Design review of the part built by this model. Coordinates are the model's own, in mm. Face numbers are marked on the shaded views. Round coordinates to 2 decimals unless told otherwise and drop trailing zeros. Loops run counter-clockwise (first coordinate to the right, second up) from the corner with the lowest first, then second, coordinate; pieces in that order, holes last. Notation, with made-up numbers: M -26.5,31.25 L -8.5,31.25 A15 ccw -8.5,50.25 Z; hole C 45,48.25 d11. An arc over 180 degrees is marked long. Use a Markdown table: item, result.
from build123d import *

# Parameters (mm, degrees)
EXTRUSION1_DEPTH = 6
HOLE1_D          = 3
HOLE2_D          = 3.2
SKETCH6_W        = 25
SKETCH6_H        = 6
EXTRUSION3_DEPTH = 10
EXTRUSION4_DEPTH = 6
FILLET1_R        = 5
SKETCH8_R        = 6.5
EXTRUSION5_DEPTH = 10


with BuildPart() as part:
    # Sketch1 → Extrusion1 (new body)
    with BuildSketch(Plane.XY):
        Polygon((35, -40), (35, 14.019237886), (20, 40), (0, 40), (0, -40), align=None)
    extrusion1 = extrude(amount=EXTRUSION1_DEPTH)

    # Mirror1: Extrusion1 across plane
    add(extrusion1.mirror(Plane(origin=(0, -8, 3), x_dir=(0, 0, 1), z_dir=(-1, 0, 0))))

    # Hole1 (through all)
    with Locations(Plane(origin=(0, 0, 0), x_dir=(-1, 0, 0), z_dir=(0, 0, -1))):
        with Locations((-6.975556847, 36), (-14.5, 15.326762343), (14.5, 15.326762343), (6.975556847, 36)):
            Hole(HOLE1_D / 2)

    # Hole2 (through all)
    with Locations(Plane.XY.offset(6)):
        with Locations((-22.1, -5.629932362), (-22.1, -15.629932362), (27.4, -15.629932362), (27.4, -5.629932362)):
            Hole(HOLE2_D / 2)

    # Sketch6 → Extrusion3 (cut)
    with BuildSketch(Plane(origin=(0, 0, 0), x_dir=(-1, 0, 0), z_dir=(0, 0, -1))):
        with Locations((0, -37)):
            Rectangle(SKETCH6_W, SKETCH6_H)
    extrude(amount=-EXTRUSION3_DEPTH, mode=Mode.SUBTRACT)

    # Sketch7 → Extrusion4 (add)
    with BuildSketch(Plane.XY.offset(6)):
        Polygon((-20, 40), (-18.267949192, 43), (18.267949192, 43), (20, 40), align=None)
    extrude(amount=-EXTRUSION4_DEPTH)

    # Fillet1
    fillet1_edges = [part.edges().sort_by_distance(p)[0] for p in [
        (-35, 14.019237886, 3),
        (-18.267949192, 43, 3),
        (18.267949192, 43, 3),
        (35, 14.019237886, 3),
    ]]
    fillet(fillet1_edges, radius=FILLET1_R)

    # Sketch8 → Extrusion5 (cut)
    with BuildSketch(Plane.XY.offset(6)):
        with Locations((-7.7, -10.629932362)):
            Circle(SKETCH8_R)
    extrude(amount=-EXTRUSION5_DEPTH, mode=Mode.SUBTRACT)


solid = part.part
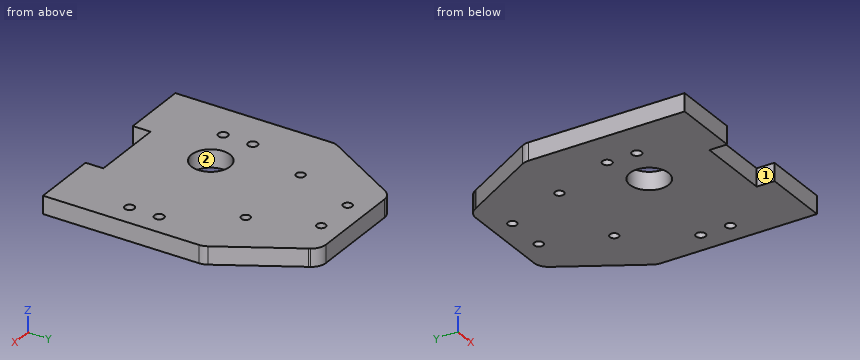
1. The part is to be moulded in two halves that separate along Y. For the marked faces 1 and 2, say which applies: pulls with the +Y half, pulls with the -Y half, needs draft (parallel to the pull), parting line crosses it, or undercut.
Check values:
| item | result |
|---|---|
| face 1 | needs draft |
| face 2 | undercut |
2. Take a section at C-C on z = 2.45. Count the separate pieces of the cut face and the enclosed holes in it, and give its area (3 significant figures).
Check values:
| item | result |
|---|---|
| separate pieces | 1 |
| enclosed holes | 9 |
| area | 4,980 mm² |
3. Take a section at B-B on x = -22. Give the boundary of the cut face in (y, z).
Check values:
| item | result |
|---|---|
| outline | M -40,0 L -17.23,0 L -17.23,6 L -40,6 Z; M -14.03,0 L -7.23,0 L -7.23,6 L -14.03,6 Z; M -4.03,0 L 36.54,0 L 36.54,6 L -4.03,6 Z |
4. Wall thickness on line 1 along X through (y, z) = (-14, 3.1); line 2 along Y through (x, z) = (-7.7, 4); line 3 along X through (y, z) = (-10, 1.85): over which ranges is each line inside the solid? List them lowest first. Write a range as from..to.
Check values:
| item | result |
|---|---|
| line 1 | x = -35..-13.26, -2.14..35 |
| line 2 | y = -34..-17.13, -4.13..34.69, 37.31..43 |
| line 3 | x = -35..-14.17, -1.23..35 |
5. Take a section at D-D on y = 36. Give the boundary of the cut face in (x, z), and give its area (3 significant figures).
Check values:
| item | result |
|---|---|
| outline | M -22.31,0 L -8.48,0 L -8.48,6 L -22.31,6 Z; M -5.48,0 L 5.48,0 L 5.48,6 L -5.48,6 Z; M 8.48,0 L 22.31,0 L 22.31,6 L 8.48,6 Z |
| area | 232 mm² |
6. Take a section at A-A on x = 14.5. Give the boundary of the cut face in (y, z), and give its area (3 significant figures).
Check values:
| item | result |
|---|---|
| outline | M -40,0 L 13.83,0 L 13.83,6 L -40,6 Z; M 16.83,0 L 43,0 L 43,6 L 16.83,6 Z |
| area | 480 mm² |
7. Insertion check: pin 1 (1.8 mm diameter, centred on x = 3.5, z = 3, fed in from -Y); pin 2 (2.5 mm diameter, centred on x = 14.5, y = 15.33, fed in from +Z). Each pin has a flat end and moves straight along its axis. Give the tip position at first contact, or say it passes through.
Check values:
| item | result |
|---|---|
| pin 1 | stops at y = -34 |
| pin 2 | passes through |
